The drawing under review shows one solid part. Ordinate dimensions are in mm from its lowest x, y, z. A direction names the side the tool comes from. Coordinates: 2 decimals unless noted, no trailing zeros. Write each loop counter-clockwise with the first axis right and the second up, starting at its lowest first coordinate (ties: lowest second). Pieces come first, ordered by that corner, then holes. Notation, with made-up numbers: (86, 81) - (122, 81) arc R7 cw to (122, 91) - close; hole circle Ø11 at (81.25, 82.5). An arc over 180 degrees is marked (long way). Use a Markdown table: item, result.
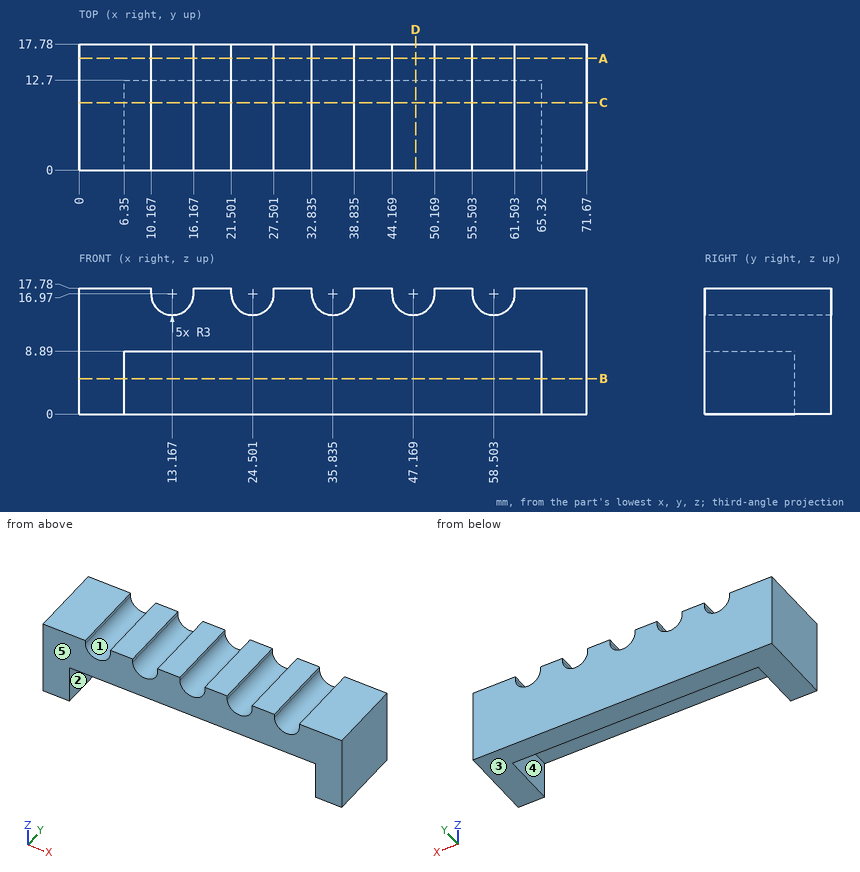
(1) Take a section at D-D on x = 47.5. Write out the cut boundary in (y, z).
Determined:
| item | result |
|---|---|
| outline | (0, 8.89) - (12.7, 8.89) - (12.7, 0) - (17.78, 0) - (17.78, 13.99) - (0, 13.99) - close |
(2) Take a section at C-C on y = 9.5. Write out the cut boundary in (x, z) (3 decimals), and give its area (3 significant figures).
Determined:
| item | result |
|---|---|
| outline | (0, 0) - (6.35, 0) - (6.35, 8.89) - (65.32, 8.89) - (65.32, 0) - (71.67, 0) - (71.67, 17.78) - (61.503, 17.78) - (61.503, 16.97) arc R3 cw to (55.503, 16.97) - (55.503, 17.78) - (50.169, 17.78) - (50.169, 16.97) arc R3 cw to (44.169, 16.97) - (44.169, 17.78) - (38.835, 17.78) - (38.835, 16.97) arc R3 cw to (32.835, 16.97) - (32.835, 17.78) - (27.501, 17.78) - (27.501, 16.97) arc R3 cw to (21.501, 16.97) - (21.501, 17.78) - (16.167, 17.78) - (16.167, 16.97) arc R3 cw to (10.167, 16.97) - (10.167, 17.78) - (0, 17.78) - close |
| area | 655 mm2 |
(3) Draft analysis for pull direction Z (two halves, no side actions). For the marked faces 1, 2 and 3, state which applies: +Z half, -Z half, draft (parallel to the pull), parting line (faces both ways), or undercut.
Determined:
| item | result |
|---|---|
| face 1 | +Z half |
| face 2 | draft |
| face 3 | -Z half |
(4) Machinability: for the marked faces 4 and 5, which of the approach directions +Z, -Z, +X, -X, +Y, -Y give a long, thin tool a straight path to every point of the face, cutting with its end or side? Answer none if there is none.
Determined:
| item | result |
|---|---|
| face 4 | -Z, -Y |
| face 5 | +Z, -Z, +X, -X, -Y |
(5) For pin 1 (1.5 mm diameter, centred on x = 34.5, y = 10.5, fed in from -Z), flat-tipped, find the tip position at first contact; note if it passes through.
Determined:
| item | result |
|---|---|
| pin 1 | z = 8.89 |
(6) For L1, parallel to X at y = 9, z = 17.25 (3 decimals); L2, parallel to X at y = 6.5, z = 7; L3, parallel to Y at x = 8, z = 7.75, list the stretches that pass through material, from the lowest coordinate up. Write a range as from..to.
Determined:
| item | result |
|---|---|
| L1 | 0..10.167, 16.167..21.501, 27.501..32.835, 38.835..44.169, 50.169..55.503, 61.503..71.67 |
| L2 | 0..6.35, 65.32..71.67 |
| L3 | 12.7..17.78 |
(7) Take a section at B-B on z = 5. Write out the cut boundary in (x, y).
Determined:
| item | result |
|---|---|
| outline | (0, 0) - (6.35, 0) - (6.35, 12.7) - (65.32, 12.7) - (65.32, 0) - (71.67, 0) - (71.67, 17.78) - (0, 17.78) - close |
(8) Take a section at A-A on y = 15.75. Write out the cut boundary in (x, z) (3 decimals).
Determined:
| item | result |
|---|---|
| outline | (0, 0) - (71.67, 0) - (71.67, 17.78) - (61.503, 17.78) - (61.503, 16.97) arc R3 cw to (55.503, 16.97) - (55.503, 17.78) - (50.169, 17.78) - (50.169, 16.97) arc R3 cw to (44.169, 16.97) - (44.169, 17.78) - (38.835, 17.78) - (38.835, 16.97) arc R3 cw to (32.835, 16.97) - (32.835, 17.78) - (27.501, 17.78) - (27.501, 16.97) arc R3 cw to (21.501, 16.97) - (21.501, 17.78) - (16.167, 17.78) - (16.167, 16.97) arc R3 cw to (10.167, 16.97) - (10.167, 17.78) - (0, 17.78) - close |
